CAD build for the part. Positions are in the model's coordinates, mm. Face numbers are marked on the shaded views. A direction names the side the tool comes from. Coordinates: 2 decimals unless noted, no trailing zeros. Order: outer loops, then holes, each group sorted by start corner. A loop starts at its lowest first (then second) coordinate and runs counter-clockwise, first axis right, second up. Notation, with made-up numbers: M 74,-2.5 L 96,-2.5 A31 cw 96,21.5 Z; hole C 74,72.5 d3. An arc over 180 degrees is marked long. One line per item, written item: value.
from build123d import *

# Parameters (mm, degrees)
SKETCH_1_R          = 2.65
EXTRUDE_1_DEPTH     = 8
SKETCH_7_W          = 8
SKETCH_7_H          = 25
EXTRUDE_2_DEPTH     = 43
SKETCH_8_W          = 8
SKETCH_8_H          = 25
EXTRUDE_3_DEPTH     = 12
SKETCH_9_R          = 4.5
CUT_EXTRUDE_1_DEPTH = 3


with BuildPart() as part:
    # 草图1 → 凸台-拉伸1 (new body)
    with BuildSketch(Plane.XY):
        Polygon((-8, 12.5), (129.3, 12.5), (129.3, -12.5), (-8, -12.5), (-9, -12.5), (-9, 12.5), align=None)
        Circle(SKETCH_1_R, mode=Mode.SUBTRACT)
    extrude(amount=EXTRUDE_1_DEPTH)

    # 草图7 → 凸台-拉伸2 (add)
    with BuildSketch(Plane(origin=(0, 0, 0), x_dir=(-1, 0, 0), z_dir=(0, 0, -1))):
        with Locations((-125.3, 0)):
            Rectangle(SKETCH_7_W, SKETCH_7_H)
    extrude(amount=EXTRUDE_2_DEPTH)

    # 草图8 → 凸台-拉伸3 (add)
    with BuildSketch(Plane.ZY.offset(-121.3)):
        with Locations((-39, 0)):
            Rectangle(SKETCH_8_W, SKETCH_8_H)
    extrude(amount=EXTRUDE_3_DEPTH)

    # 草图9 → 切除-拉伸1 (cut)
    with BuildSketch(Plane.XY.offset(8)):
        Circle(SKETCH_9_R)
    extrude(amount=-CUT_EXTRUDE_1_DEPTH, mode=Mode.SUBTRACT)


solid = part.part
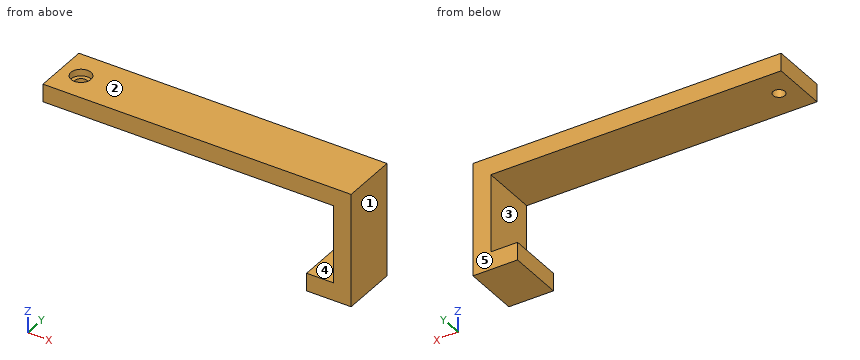
Q1. Slice it at A-A (x = 0). List the corners of the cut face in (y, z), plus the area to 4 significant figures.
Recorded:
outline: M -12.5,0 L -2.65,0 L -2.65,5 L -4.5,5 L -4.5,8 L -12.5,8 Z; M 2.65,0 L 12.5,0 L 12.5,8 L 4.5,8 L 4.5,5 L 2.65,5 Z
area: 146.5 mm^2
Q2. Pin check, flat tips, straight feed: pin 1 Ø12 at (x, y) = (10.5, -8.5) entering from -Z; pin 2 Ø7 at (x, y) = (-2, -2) entering from +Z; pin 3 Ø7.5 at (y, z) = (-1.5, -17.5) entering from -X; pin 4 Ø4 at (y, z) = (0, -40) entering from -X. Stop position of each tip, or through.
Recorded:
pin 1: stops at z = 0
pin 2: stops at z = 8
pin 3: stops at x = 121.3
pin 4: stops at x = 109.3
Q3. Mould opens along Z. For the marked faces 1, 2 and 3 say: released by +Z, released by -Z, zero draft, split by the parting line, or undercut.
Recorded:
face 1: zero draft
face 2: released by +Z
face 3: undercut
Q4. Slice it at D-D (z = -2). List the corners of the cut face in (x, y).
Recorded:
outline: M 121.3,-12.5 L 129.3,-12.5 L 129.3,12.5 L 121.3,12.5 Z
Q5. Which spindle directions (+Z, -Z, +X, -X, +Y, -Y) get a long thin tool onto all of the face, cutting with end or side? Do the marked faces 4 and 5. Say none if no direction does.
Recorded:
face 4: -X, +Y, -Y
face 5: +Z, -Z, +X, -X, +Y
Q6. Slice it at B-B (y = 0). List the corners of the cut face in (x, z), plus the area to 3 significant figures.
Recorded:
outline: M -9,0 L -2.65,0 L -2.65,5 L -4.5,5 L -4.5,8 L -9,8 Z; M 2.65,0 L 121.3,0 L 121.3,-35 L 109.3,-35 L 109.3,-43 L 129.3,-43 L 129.3,8 L 4.5,8 L 4.5,5 L 2.65,5 Z
area: 1,490 mm^2
Q7. Slice it at C-C (y = -6.5). List the corners of the cut face in (x, z).
Recorded:
outline: M -9,0 L 121.3,0 L 121.3,-35 L 109.3,-35 L 109.3,-43 L 129.3,-43 L 129.3,8 L -9,8 Z
Q8. Drill centre lines: line 1 along Z through (x, y) = (115, 6.5); line 2 along Y through (x, z) = (0, 3); line 3 along X through (y, z) = (0, 2.3). Where is each one in solid material? Low to high.
Recorded:
line 1: z = -43 to -35, 0 to 8
line 2: y = -12.5 to -2.65, 2.65 to 12.5
line 3: x = -9 to -2.65, 2.65 to 129.3
